Source: CAD feature listing. Evaluate the final solid. Frame: model axes, mm. A direction names the side the tool comes from. Round coordinates to 2 decimals unless told otherwise and drop trailing zeros. Loops run counter-clockwise (first coordinate to the right, second up) from the corner with the lowest first, then second, coordinate; pieces in that order, holes last. Notation, with made-up numbers: (68.5, 10) -> (92.5, 10) arc R26 cw to (92.5, 46) -> close; hole circle Ø4 at (20, 3). An arc over 180 degrees is marked (long way). Put each result on its own line as item: value. Start each with the question number.
1. Cut plane C-C (x = -5.75). Return the cut outline in (y, z), then the cut area to 3 significant figures.
2. Contact query for flat-ended pins moving along their axis: pin 1 (1.4 mm diameter, centred on y = 3, z = -1, fed in from -X); pin 2 (2 mm diameter, centred on x = -5, y = 3.5, fed in from +Z); pin 3 (1.6 mm diameter, centred on y = -1, z = -5.5, fed in from +X). Output: stop coordinate, or through.
3. Draft query along Z for faces 1 (the cylindrical face through (7, 3.3, -7.4)), 2 (the flat face through (0.06, -1.56, -13.74)), 3 (the flat face through (-4.5, 3, -14)). Return one class per face: pulls with the +Z half, pulls with the -Z half, needs draft (parallel to the pull), parting line crosses it, or undercut.
4. Material intervals for L1, parallel to X at y = 1.25, z = -13.25; L2, parallel to Z at x = 0.75, y = 5.5; L3, parallel to X at y = 4.5, z = -12, sorted ascending.
5. Set-up query: faces 4 (the flat face through (-0.06, -1.73, -6.81)), 5 (the flat face through (0, 6.2, 2)), 6 (the flat face through (0, 5.9, 2)), 7 (the flat face through (0, -1.3, 2)), 8 (the flat face through (4.5, 3, -14)). Return all of +Z, -Z, +X, -X, +Y, -Y with unobstructed straight access to the full face (end or side cutting, diameter ignored); none if empty.
6. Cut plane A-A (y = -0.25). Return the cut outline in (x, z), then the cut area to 3 significant figures.
7. Cut plane B-B (z = -7). Return the cut outline in (x, y).
Autodesk Inventor part; units mm, degrees
ref_plane "作業平面1" through (-4.5, -2.3, -0.3) normal (0, 0.9962, 0.0872) x (1, 0, 0)
ref_plane "作業平面2" through (4.5, -0.8681, -13.2244) normal (0, -0.8387, 0.5446) x (-1, 0, 0)
ref_plane "作業平面3" through (0, 6.2, 0) normal (0, 1, 0) x (1, 0, 0)
sketch "スケッチ1" plane through (0, 0, 0) normal (0, 1, 0) x (-1, 0, 0)
  line L0 (4.5, -0.3) -> (-4.5, -0.3)
  line L1 (-4.5, -0.3) -> (-4.5, 0)
  line L2 (-4.5, 0) -> (4.5, 0)
  line L3 (4.5, 0) -> (4.5, -0.3)
  line L4 (9.7545, -2) -> (-9.7545, -2) construction
  line L5 (0, -25.3634) -> (0, 2.8638) construction
  circle A0 centre (0, -7.3619) radius 7
  circle A1 centre (0, -7.3619) radius 6.7
  line L6 (4.5, -0.3) -> (4.5, -2)
  line L7 (4.2, -0.3) -> (4.2, -2.1417)
  line L8 (-4.5, -0.3) -> (-4.5, -2)
  line L9 (-4.2, -0.3) -> (-4.2, -2.1417)
  line L10 (9.7545, -15) -> (-9.7545, -15) construction
  line L11 (4.5, -12.7238) -> (4.5, -15)
  line L12 (4.5, -15) -> (4.2, -15)
  line L13 (4.2, -12.5821) -> (4.2, -15)
  line L14 (-4.5, -12.7238) -> (-4.5, -15)
  line L15 (-4.5, -15) -> (-4.2, -15)
  line L16 (-4.2, -15) -> (-4.2, -12.5821)
  point P0 (0, 0)
  point P1 (0, 0)
  point P2 (0, -2)
  point P3 (0, -15)
  dimension "d0" = 9
  dimension "THIN" = 0.3
  dimension "d2" = 2
  dimension "d3" = 14
  dimension "d5" = 0.3
  dimension "d6" = 0.3
  dimension "d7" = 0.3
  dimension "d8" = 15
extrude "押し出し1" add sketch "スケッチ1" along normal blind 6.7 contours L6 A0 L7 L0 | L0 L1 L2 L3 | A0 L13 A1 L7 | L9 A0 L8 L0 | L9 A1 L16 A0 | L11 L12 L13 A0 | A0 L16 L15 L14
sketch "スケッチ2" plane through (0, 0, 0) normal (0, -1, 0) x (1, 0, 0)
  line L0 (4.5, 0) -> (4.5, -2)
  line L1 (-4.5, -2) -> (-4.5, 0)
  line L2 (4.5, 0) -> (-4.5, 0)
  line L3 (-4.5, 0) -> (-4.5, -0.3)
  line L4 (-4.5, -0.3) -> (4.5, -0.3)
  line L5 (4.5, -0.3) -> (4.5, 0)
  line L6 (4.2, -0.3) -> (-4.2, -0.3)
  point P0 (0, 0)
  point P1 (4.5, -0.3)
extrude "押し出し2" add sketch "スケッチ2" along normal blind 2.3
ref_plane "作業平面1" through (-4.5, -2.3, -0.3) normal (0, 0.9962, 0.0872) x (1, 0, 0)
sketch "スケッチ3" plane through (-4.5, -2.3, -0.3) normal (0, 0.9962, 0.0872) x (1, 0, 0)
  line L0 (0, 0) -> (9, 0)
  line L1 (9, 0) -> (0, 0)
  line L2 (0, 0) -> (0, 13)
  line L3 (0, 13) -> (9, 13)
  line L4 (9, 13) -> (9, 0)
  point P0 (4.5, -0.0984)
  dimension "d14" = 13
extrude "押し出し3" add sketch "スケッチ3" along normal blind 0.3
ref_plane "作業平面2" through (4.5, -0.8681, -13.2244) normal (0, -0.8387, 0.5446) x (-1, 0, 0)
sketch "スケッチ4" plane through (4.5, -0.8681, -13.2244) normal (0, -0.8387, 0.5446) x (-1, 0, 0)
  line L0 (9, 0) -> (9, -10.2235)
  line L1 (9, 0) -> (0, 0)
  line L2 (0, 0) -> (0, 1.5)
  line L3 (0, 1.5) -> (9, 1.5)
  line L4 (9, 1.5) -> (9, 0)
  point P0 (4.5, -11.5637)
  dimension "d18" = 1.5
extrude "押し出し4" add sketch "スケッチ4" along normal blind 0.3
sketch "スケッチ5" plane through (4.2, 6.7, -0.3) normal (0, 0, -1) x (-1, 0, 0)
  line L0 (5.95, -2) -> (2.45, -2)
  line L1 (2.45, -2) -> (2.45, -7.7)
  line L2 (2.45, -7.7) -> (5.95, -7.7)
  line L3 (5.95, -7.7) -> (5.95, -2)
  line L4 (0, 0) -> (8.4, 0)
  point P0 (4.2, -6.7)
  point P1 (4.2, -7.7)
  dimension "d21" = 2
  dimension "d22" = 3.5
  dimension "d23" = 5.7
extrude "押し出し5" cut sketch "スケッチ5" against normal through all
sketch "スケッチ7" plane through (-1.75, -1, -0.3) normal (0, 1, 0) x (1, 0, 0)
  line L0 (3.5, -0.3) -> (0, -0.3)
  line L1 (1, -0.3) -> (2.5, -0.3)
  line L2 (2.5, -0.3) -> (2.5, -4.7)
  line L3 (2.5, -4.7) -> (1, -4.7)
  line L4 (1, -4.7) -> (1, -0.3)
  point P0 (1.75, -0.3)
  point P1 (1.75, -0.3)
  dimension "d30" = 1.5
  dimension "d31" = 4.4
extrude "押し出し7" add sketch "スケッチ7" against normal blind 0.3
ref_plane "作業平面3" through (0, 6.2, 0) normal (0, 1, 0) x (1, 0, 0)
sketch "スケッチ8" plane through (0, 6.2, 0) normal (0, 1, 0) x (1, 0, 0)
  line L0 (4.5, 0) -> (-4.5, 0)
  line L1 (-0.75, 0) -> (0.75, 0)
  line L2 (0.75, 0) -> (0.75, -4.4)
  line L3 (0.75, -4.4) -> (-0.75, -4.4)
  line L4 (-0.75, -4.4) -> (-0.75, 0)
  line L5 (-4.5, 0) -> (4.5, 0)
  point P0 (0, 0)
  point P1 (0, -4.4)
  point P2 (0, 0)
  dimension "d35" = 1.5
  dimension "d36" = 4.4
extrude "押し出し8" add sketch "スケッチ8" against normal blind 0.3
equation "\"d5\" = THIN"
equation "\"d6\" = THIN"
equation "\"d7\" = THIN"
equation "\"d15\" = THIN"
equation "\"d19\" = THIN"
equation "\"d32\" = THIN"
equation "\"d37\" = THIN"
properties part number "AA-Cell-Holder"
Solution:
1. outline: (0, -11.35) -> (6.7, -11.35) -> (6.7, -10.8) -> (0, -10.8) -> close; (0, -3.92) -> (6.7, -3.92) -> (6.7, -3.37) -> (0, -3.37) -> close
1. area: 7.41 mm^2
2. pin 1: stops at x = -4.5
2. pin 2: stops at z = 0
2. pin 3: stops at x = 4.5
3. face 1: parting line crosses it
3. face 2: undercut
3. face 3: needs draft
4. L1: x = -4.5 to -4.2, 4.2 to 4.5
4. L2: z = -0.3 to 0
4. L3: x = -5.24 to -4.84, 4.84 to 5.24
5. face 4: +X, -X, -Y
5. face 5: +Z, +X, -X, +Y
5. face 6: +Z, +X, -X
5. face 7: +Z, +X, -X, -Y
5. face 8: -Z, +X, +Y, -Y
6. outline: (-4.5, -0.3) -> (-1.75, -0.3) -> (-1.75, 0) -> (-4.5, 0) -> close; (1.75, -0.3) -> (4.5, -0.3) -> (4.5, 0) -> (1.75, 0) -> close
6. area: 1.65 mm^2
7. outline: (-6.99, 0) -> (-6.69, 0) -> (-6.69, 6.7) -> (-6.99, 6.7) -> close; (-4.5, -1.71) -> (4.5, -1.71) -> (4.5, -1.41) -> (-4.5, -1.41) -> close; (6.69, 0) -> (6.99, 0) -> (6.99, 6.7) -> (6.69, 6.7) -> close
